```python
from build123d import *

# Parameters (mm, degrees)
SKETCH1_R           = 3
BOSS_EXTRUDE1_DEPTH = 12
SKETCH2_R           = 3.5
BOSS_EXTRUDE2_DEPTH = 1
SKETCH3_R           = 8
BOSS_EXTRUDE3_DEPTH = 44.4
SKETCH4_R           = 1
CUT_EXTRUDE1_DEPTH  = 3


with BuildPart() as part:
    # Sketch1 → Boss-Extrude1 (new body)
    with BuildSketch(Plane.XY):
        Circle(SKETCH1_R)
    extrude(amount=BOSS_EXTRUDE1_DEPTH)

    # Sketch2 → Boss-Extrude2 (add)
    with BuildSketch(Plane(origin=(0, 0, 0), x_dir=(-1, 0, 0), z_dir=(0, 0, -1))):
        Circle(SKETCH2_R)
    extrude(amount=BOSS_EXTRUDE2_DEPTH)

    # Sketch3 → Boss-Extrude3 (add)
    with BuildSketch(Plane(origin=(0, 0, -1), x_dir=(-1, 0, 0), z_dir=(0, 0, -1))):
        Circle(SKETCH3_R)
    extrude(amount=BOSS_EXTRUDE3_DEPTH)

    # Sketch4 → Cut-Extrude1 (cut)
    with BuildSketch(Plane.XY.offset(-1)):
        with Locations((0, 5.5)):
            Circle(SKETCH4_R)
        with Locations((0, -5.5)):
            Circle(SKETCH4_R)
    extrude(amount=-CUT_EXTRUDE1_DEPTH, mode=Mode.SUBTRACT)


solid = part.part
```
Model file for the job. Use its own axes, mm. A direction names the side the tool comes from. Round coordinates to 2 decimals unless told otherwise and drop trailing zeros. Loops run counter-clockwise (first coordinate to the right, second up) from the corner with the lowest first, then second, coordinate; pieces in that order, holes last. Notation, with made-up numbers: M -10,34.5 L 31,34.5 A24 ccw 31,66.5 Z; hole C 43,-4 d2. An arc over 180 degrees is marked long. Put each result on its own line as item: value. Start each with the question number.
Item 1: Mould opens along Y. For faces 1 (the face through (0, 0, 12)), 2 (the face through (1.73, -7.81, -22.89)), 3 (the face through (0, 6, -4)) say: released by +Y, released by -Y, zero draft, split by the parting line, or undercut.
Item 2: Cut at B-B (x = -0.5). List the corners of the cut face in (y, z), then the cut area to 3 significant figures.
Item 3: Drop flat-ended pins along their axis: P1, Ø6, axis at y = 2.5, z = 4, coming from the -X side; P2, Ø2, axis at x = -0.5, y = 5.5, coming from the +Z side; P3, Ø2, axis at x = 1, y = 4, coming from the +Z side; P4, Ø8, axis at x = 4, z = -36, coming from the -Y side. Give the stop position or say it passes through.
Item 4: Cut at D-D (y = -5). List the corners of the cut face in (x, z) (3 decimals).
Item 5: 3-axis set-ups, long thin cutter, end or side, ignore diameter. For faces 4 (the face through (0, -5, -4)), 5 (the face through (0, 0, -45.4)): which of +Z, -Z, +X, -X, +Y, -Y reach the whole face in a straight line?
Item 6: Cut at C-C (z = -12.5). List the corners of the cut face in (x, y), then the cut area to 3 significant figures.
Item 7: Drill centre lines: line 1 along Y through (x, z) = (0, -1.65); line 2 along Z through (x, y) = (0, 6.25); line 3 along Z through (x, y) = (-2.25, 7.25). Where is each one in solid material? Low to high.
Item 8: Cut at A-A (y = 0). List the corners of the cut face in (x, z), then the cut area to 3 significant figures.
Answer block:
1. face 1: zero draft
1. face 2: split by the parting line
1. face 3: undercut
2. outline: M -7.98,-45.4 L 7.98,-45.4 L 7.98,-1 L 6.37,-1 L 6.37,-4 L 4.63,-4 L 4.63,-1 L 3.46,-1 L 3.46,0 L 2.96,0 L 2.96,12 L -2.96,12 L -2.96,0 L -3.46,0 L -3.46,-1 L -4.63,-1 L -4.63,-4 L -6.37,-4 L -6.37,-1 L -7.98,-1 Z
2. area: 777 mm2
3. P1: x = -3
3. P2: z = -1
3. P3: z = 0
3. P4: y = -8
4. outline: M -6.245,-45.4 L 6.245,-45.4 L 6.245,-1 L 0.866,-1 L 0.866,-4 L -0.866,-4 L -0.866,-1 L -6.245,-1 Z
5. face 4: +Z
5. face 5: -Z, +X, -X, +Y, -Y
6. outline: C 0,0 d16
6. area: 201 mm2
7. line 1: -8 to -6.5, -4.5 to 4.5, 6.5 to 8
7. line 2: -45.4 to -4
7. line 3: -45.4 to -1
8. outline: M -8,-45.4 L 8,-45.4 L 8,-1 L 3.5,-1 L 3.5,0 L 3,0 L 3,12 L -3,12 L -3,0 L -3.5,0 L -3.5,-1 L -8,-1 Z
8. area: 789 mm2
